Source: CAD feature listing. Evaluate the final solid. Frame: model axes, mm. A direction names the side the tool comes from. Give positions to 0.01 mm unless a question says otherwise; leave off trailing zeros. Order: outer loops, then holes, each group sorted by start corner. A loop starts at its lowest first (then second) coordinate and runs counter-clockwise, first axis right, second up. Notation, with made-up numbers: M 5,-31 L 17,-31 A21 cw 17,-9 Z; hole C -3.5,17.25 d6. An arc over 180 degrees is marked long. Answer in a Markdown table with one row per item. Add a question column.
(1) Section query D-D, the plane y = -16. Return loops of the section in (x, z).
(2) Section query A-A, the plane y = 0. Return loops of the section in (x, z).
(3) Material intervals for line 1 along X through (y, z) = (22, 8); line 2 along X through (y, z) = (8, 8); line 3 along Z through (x, y) = (60, -19.5), sorted ascending.
(4) Section query C-C, the plane x = 95. Return loops of the section in (y, z).
(5) Set-up query: faces 1 (the face through (25.73, -5.27, -16.736)), 2 (the face through (110.26, 5.34, 6.96)), 3 (the face through (131.286, 0, 0)). Return all of +Z, -Z, +X, -X, +Y, -Y with unobstructed straight access to the full face (end or side cutting, diameter ignored); none if empty.
(6) Pin query (flat end, axial travel): P1, Ø6, axis at y = -22.5, z = -18.5, coming from the +X side; P2, Ø1.5, axis at x = 51, y = -19, coming from the -Z side; P3, Ø12, axis at x = 87.5, z = -21.5, coming from the -Y side; P4, Ø4, axis at y = -19, z = -0.5, coming from the -X side. Return the tip coordinate at first contact, or that it passes through.
from build123d import *


with BuildPart() as part:
    # Skica1 → Rotovat1 (revolve)
    with BuildSketch(Plane.XY, mode=Mode.PRIVATE) as rotovat1_sk:
        Polygon((0, 0), (0, 17.545735619), (50.749167087, 17.545735619), (50.749167087, 28.852573965), (88.636993826, 28.852573965), (88.636993826, 8.772867809), (131.285594605, 8.772867809), (131.285594605, 0), align=None)
    revolve(rotovat1_sk.sketch.rotate(Axis((131.285594605, 0, 0), (-1, 0, 0)), 90), axis=Axis((131.285594605, 0, 0), (-1, 0, 0)))  # turned: the seam where the file's is


solid = part.part
Values follow:
| question | item | result |
|---|---|---|
| 1 | outline | M 0,-7.2 L 50.75,-7.2 L 50.75,-24.01 L 88.64,-24.01 L 88.64,24.01 L 50.75,24.01 L 50.75,7.2 L 0,7.2 Z |
| 2 | outline | M 0,-17.55 L 50.75,-17.55 L 50.75,-28.85 L 88.64,-28.85 L 88.64,-8.77 L 131.29,-8.77 L 131.29,8.77 L 88.64,8.77 L 88.64,28.85 L 50.75,28.85 L 50.75,17.55 L 0,17.55 Z |
| 3 | line 1 | x = 50.75 to 88.64 |
| 3 | line 2 | x = 0 to 88.64 |
| 3 | line 3 | z = -21.27 to 21.27 |
| 4 | outline | C 0,0 d17.55 |
| 5 | face 1 | -X |
| 5 | face 2 | +X |
| 5 | face 3 | +Z, -Z, +X, +Y, -Y |
| 6 | P1 | stops at x = 88.64 |
| 6 | P2 | stops at z = -22.35 |
| 6 | P3 | stops at y = -24.34 |
| 6 | P4 | stops at x = 0 |
